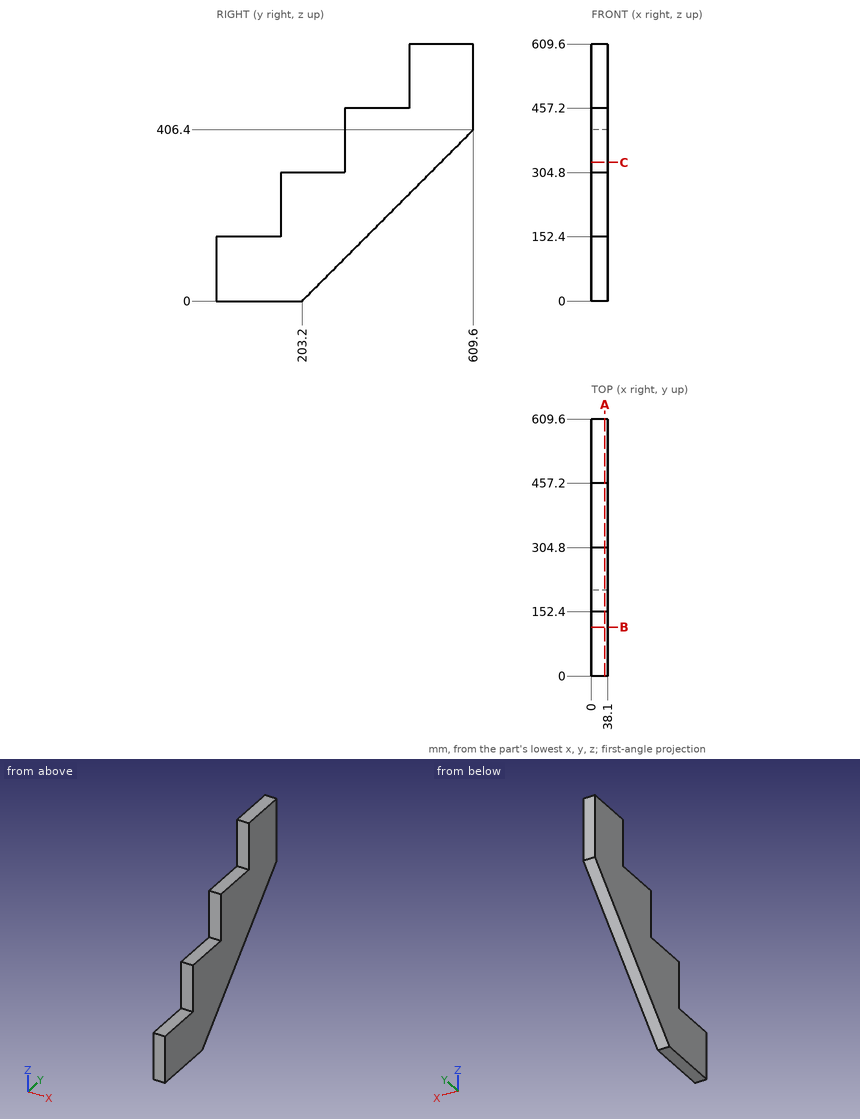
Input: dimensioned drawing with shaded views. Units: mm. Origin: part minimum x, y, z. Give positions to 0.01 mm unless a question says otherwise; leave off trailing zeros. Order: outer loops, then holes, each group sorted by start corner. A loop starts at its lowest first (then second) coordinate and runs counter-clockwise, first axis right, second up.
(1) Section query A-A (x = 31.5). Return the cut outline in (y, z).
(2) Section query B-B (y = 116). Return the cut outline in (x, z).
(3) Material intervals for line 1 along Z through (x, y) = (10, 151); line 2 along Y through (x, z) = (27, 529.5); line 3 along Z through (x, y) = (14.5, 192), sorted ascending.
(4) Contact query for flat-ended pins moving along their axis: P1, Ø12, axis at x = 23, y = 518.5, coming from the -Z side; P2, Ø10, axis at x = 15.5, y = 179, coming from the +Z side; P3, Ø19, axis at x = 22.5, z = 525.5, coming from the -Y side. Output: stop coordinate, or through.
(5) Section query C-C (z = 329). Return the cut outline in (x, y).
Outcome:
1. outline: (0, 0) - (203.2, 0) - (609.6, 406.4) - (609.6, 609.6) - (457.2, 609.6) - (457.2, 457.2) - (304.8, 457.2) - (304.8, 304.8) - (152.4, 304.8) - (152.4, 152.4) - (0, 152.4) - close
2. outline: (0, 0) - (38.1, 0) - (38.1, 152.4) - (0, 152.4) - close
3. line 1: z = 0 to 152.4
3. line 2: y = 457.2 to 609.6
3. line 3: z = 0 to 304.8
4. P1: stops at z = 309.3
4. P2: stops at z = 304.8
4. P3: stops at y = 457.2
5. outline: (0, 304.8) - (38.1, 304.8) - (38.1, 532.2) - (0, 532.2) - close
